Autodesk Inventor part; units mm, degrees
ref_plane "YZ Plane" through (0, 0, 0) normal (1, 0, 0) x (0, 1, 0)
ref_plane "XZ Plane" through (0, 0, 0) normal (0, 1, 0) x (-1, 0, 0)
ref_plane "XY Plane" through (0, 0, 0) normal (0, 0, 1) x (1, 0, 0)
sketch "Sketch1" plane through (0, 0, 0) normal (0, 1, 0) x (-1, 0, 0)
  line L0 (0, 0) -> (31, 0)
  line L1 (31, 0) -> (31, 4)
  line L2 (32, 5) -> (49, 5)
  line L3 (50, 4) -> (50, 0)
  line L4 (50, 0) -> (68, 0)
  line L5 (68, -52) -> (68, -85)
  line L6 (69, -86) -> (70, -86)
  line L7 (71, -87) -> (71, -272.1)
  line L8 (71, -272.1) -> (72.1718, -272.1)
  line L9 (72.8789, -272.3929) -> (74.7071, -274.2211)
  line L10 (75, -274.9282) -> (75, -284.1718)
  line L11 (74.7071, -284.8789) -> (72.8789, -286.7071)
  line L12 (72.1718, -287) -> (71, -287)
  line L13 (71, -287) -> (71, -293.6)
  line L14 (71, -293.6) -> (-26.8, -293.6)
  line L15 (-29.8, -290.6) -> (-29.8, -286)
  line L16 (0, 0) -> (0, 4)
  line L17 (-1, 5) -> (-18, 5)
  line L18 (-19, 4) -> (-19, 0)
  line L19 (-19, 0) -> (-24.8, 0)
  line L20 (-29.8, -5) -> (-29.8, -8.5)
  line L21 (-29.8, -8.5) -> (-37.8, -8.5)
  line L22 (-40.8, -11.5) -> (-40.8, -19.5)
  line L23 (-37.8, -22.5) -> (-7.9, -22.5)
  line L24 (-6.9, -23.5) -> (-6.9, -254)
  line L25 (-7.9, -255) -> (-26.8, -255)
  line L26 (-29.8, -258) -> (-29.8, -272)
  line L27 (-29.8, -272) -> (-37.8, -272)
  line L28 (-40.8, -275) -> (-40.8, -283)
  line L29 (-37.8, -286) -> (-29.8, -286)
  circle A0 centre (53.1, -11) radius 4
  circle A1 centre (-11.9, -11) radius 4
  circle A2 centre (53.1, -275) radius 4
  circle A3 centre (-11.9, -275) radius 4
  line L30 (69, -51) -> (70, -51)
  arc A4 (-18, 5) -> (-19, 4) centre (-18, 4) ccw
  arc A5 (0, 4) -> (-1, 5) centre (-1, 4) ccw
  arc A6 (32, 5) -> (31, 4) centre (32, 4) ccw
  arc A7 (50, 4) -> (49, 5) centre (49, 4) ccw
  arc A8 (-24.8, 0) -> (-29.8, -5) centre (-24.8, -5) ccw
  arc A9 (-7.9, -255) -> (-6.9, -254) centre (-7.9, -254) ccw
  arc A10 (-26.8, -255) -> (-29.8, -258) centre (-26.8, -258) ccw
  arc A11 (-37.8, -272) -> (-40.8, -275) centre (-37.8, -275) ccw
  arc A12 (-40.8, -283) -> (-37.8, -286) centre (-37.8, -283) ccw
  arc A13 (-40.8, -19.5) -> (-37.8, -22.5) centre (-37.8, -19.5) ccw
  arc A14 (-37.8, -8.5) -> (-40.8, -11.5) centre (-37.8, -11.5) ccw
  arc A15 (72.8789, -272.3929) -> (72.1718, -272.1) centre (72.1718, -273.1) ccw
  arc A16 (75, -274.9282) -> (74.7071, -274.2211) centre (74, -274.9282) ccw
  arc A17 (74.7071, -284.8789) -> (75, -284.1718) centre (74, -284.1718) ccw
  arc A18 (72.1718, -287) -> (72.8789, -286.7071) centre (72.1718, -286) ccw
  line L31 (71, -9.1) -> (72.1718, -9.1)
  line L32 (72.8789, -9.3929) -> (74.7071, -11.2211)
  line L33 (75, -11.9282) -> (75, -21.1718)
  line L34 (74.7071, -21.8789) -> (72.8789, -23.7071)
  line L35 (72.1718, -24) -> (71, -24)
  arc A19 (72.8789, -9.3929) -> (72.1718, -9.1) centre (72.1718, -10.1) ccw
  arc A20 (75, -11.9282) -> (74.7071, -11.2211) centre (74, -11.9282) ccw
  arc A21 (74.7071, -21.8789) -> (75, -21.1718) centre (74, -21.1718) ccw
  arc A22 (72.1718, -24) -> (72.8789, -23.7071) centre (72.1718, -23) ccw
  line L36 (71, -36.1) -> (72.1718, -36.1)
  line L37 (72.8789, -36.3929) -> (74.7071, -38.2211)
  line L38 (75, -38.9282) -> (75, -48.1718)
  line L39 (74.7071, -48.8789) -> (72.8789, -50.7071)
  line L40 (72.1718, -51) -> (71, -51)
  arc A23 (72.8789, -36.3929) -> (72.1718, -36.1) centre (72.1718, -37.1) ccw
  arc A24 (75, -38.9282) -> (74.7071, -38.2211) centre (74, -38.9282) ccw
  arc A25 (74.7071, -48.8789) -> (75, -48.1718) centre (74, -48.1718) ccw
  arc A26 (72.1718, -51) -> (72.8789, -50.7071) centre (72.1718, -50) ccw
  line L41 (71, -9.1) -> (71, -3)
  line L42 (71, -24) -> (71, -36.1)
  arc A27 (69, -51) -> (68, -52) centre (69, -52) ccw
  arc A28 (68, -85) -> (69, -86) centre (69, -85) ccw
  arc A29 (71, -87) -> (70, -86) centre (70, -87) ccw
  line L43 (71, -51) -> (70, -51)
  arc A30 (71, -3) -> (68, 0) centre (68, -3) ccw
  arc A31 (-6.9, -23.5) -> (-7.9, -22.5) centre (-7.9, -23.5) ccw
  arc A32 (-29.8, -290.6) -> (-26.8, -293.6) centre (-26.8, -290.6) ccw
  circle A33 centre (-36.8, -15.5) radius 2.15
  circle A34 centre (-36.8, -279) radius 2.15
  circle A35 centre (20.6, -6.5) radius 2.5
  point P0 (31, 5)
  point P1 (50, 5)
  point P2 (71, 0)
  point P3 (68, -86)
  point P4 (71, -86)
  point P5 (72.586, -272.1)
  point P6 (72.586, -287)
  point P7 (0, 5)
  point P8 (59, 0)
  point P9 (50, 2)
  point P10 (71, -5)
  point P11 (-22.85, -22.5)
  point P12 (-33.8, -8.5)
  point P13 (71.5859, -287)
  point P14 (71.8793, -10)
  point P15 (69.5, -51)
  point P16 (-21.9, 0)
  point P17 (71.5859, -24)
  point P18 (71.5859, -51)
  point P19 (69.5, -86)
  point P20 (-29.8, -6.75)
  point P21 (40.5, 5)
  dimension "d0" = 90
  dimension "d1" = 31
  dimension "d3" = 19
  dimension "d4" = 19
  dimension "d8" = 14
  dimension "d10" = 0
  dimension "d11" = 8
  dimension "d12" = 11
  dimension "d13" = 8
  dimension "d14" = 65
  dimension "d15" = 8
  dimension "d16" = 8
  dimension "d17" = 264
  dimension "d18" = 264
  dimension "d21" = 3
  dimension "d24" = 51
  dimension "d25" = 5
  dimension "d26" = 5
  dimension "d27" = 1
  dimension "d28" = 5
  dimension "d30" = 77.9
  dimension "d32" = 1
  dimension "d33" = 3
  dimension "d34" = 17
  dimension "d35" = 14
  dimension "d36" = 11
  dimension "d37" = 3
  dimension "d38" = 22.5
  dimension "d39" = 33.9
  dimension "d40" = 3
  dimension "d41" = 11
  dimension "d42" = 4
  dimension "d43" = 14.9
  dimension "d44" = 6.6
  dimension "d45" = 1.586
  dimension "d46" = 135
  dimension "d47" = 1.586
  dimension "d48" = 135
  dimension "d49" = 1
  dimension "d50" = 14.9
  dimension "d51" = 135
  dimension "d52" = 135
  dimension "d53" = 1
  dimension "d54" = 14.9
  dimension "d55" = 135
  dimension "d56" = 135
  dimension "d57" = 1
  dimension "d58" = 9.1
  dimension "d59" = 12.1
  dimension "d61" = 1
  dimension "d62" = 35
  dimension "d63" = 100.8
  dimension "d64" = 38.6
  dimension "d67" = 3
  dimension "d68" = 1
  dimension "d69" = 3
  dimension "d70" = 232.5
  dimension "d71" = 27.5
  dimension "d74" = 293.6
  dimension "d75" = 185.1
  dimension "d76" = 4.3
  dimension "d77" = 4
  dimension "d78" = 7
  dimension "d79" = 4
extrude "Extrusion1" add sketch "Sketch1" along normal blind 5 contours L0 L1 A6 L2 A7 L3 L4 A30 L41 L31 A19 L32 A20 L33 A21 L34 A22 L35 L42 L36 A23 L37 A24 L38 A25 L39 A26 L40 L43 L30 A27 L5 A28 L6 A29 L7 L8 A15 L9 A16 L10 A17 L11 A18 L12 L13 L14 A32 L15 L29 A12 L28 A11 L27 L26 A10 L25 A9 L24 A31 L23 A13 L22 A14 L21 L20 A8 L19 L18 A4 L17 A5 L16 | A33 | A34 | A35
extrude "Extrusion2" cut sketch "Sketch1" along normal blind 5 contours A33 | A34 | A35
fillet "Fillet1" radius 3 1 edges at (-71, 2.5, -293.6)
thread "Thread1"
thread "Thread2"
thread "Thread3"
thread "Thread4"
properties part number "21-30-220-B2"
The listing builds one solid part. Answer for the finished solid, in the listing's coordinates (mm). A direction names the side the tool comes from. Coordinates: 2 decimals unless noted, no trailing zeros. Loops run counter-clockwise (first coordinate to the right, second up) from the corner with the lowest first, then second, coordinate; pieces in that order, holes last.
1) Determine the mould class of faces 1 (the face through (22, 2, 0)), 2 (the face through (34, 2, -286)), 3 (the face through (10.054, 2.465, -271.451)) for opening direction Z: pulls with the +Z half, pulls with the -Z half, needs draft (parallel to the pull), parting line crosses it, or undercut.
2) Flat-ended cylindrical pins translate along their axes: pin 1 Ø1.5 at (y, z) = (2.5, -33) entering from -X; pin 2 Ø10 at (x, z) = (16.5, -40.5) entering from +Y; pin 3 Ø0.8 at (x, y) = (-69.5, 3) entering from +Z; pin 4 Ø0.9 at (x, y) = (-71.5, 2.5) entering from -Z. Find the tip coordinate at first contact, or state that the pin passes through.
3) Find section A-A on x = -53.1. Write down the section's boundary in (y, z), then the cut area to 3 significant figures.
4) Find section C-C on y = 1.8. Give the number of separate pieces and of enclosed holes in the cut face, then the cut area to 3 significant figures.
5) A tool of negligible diameter and unlimited length cuts with its end or side. For faces 4 (the face through (34, 2, -272)), 5 (the face through (-52.233, 2.465, -271.095)), 6 (the face through (40.8, 2, -15)), 7 (the face through (-71, 2, -30)), 8 (the face through (-71, 2, -6)), from which of +Z, -Z, +X, -X, +Y, -Y can it reach the whole face along a straight path? Write none if from no direction.
6) Find section B-B on z = -212. Write down the section's boundary in (x, y).
7) Find the intervals of material crossed by L1, parallel to Z at x = 36.8, y = 3.75; L2, parallel to Z at x = -53.1, y = 3.75; L3, parallel to X at y = 2, z = -275, in increasing order.
Values:
1. face 1: pulls with the +Z half
1. face 2: pulls with the -Z half
1. face 3: undercut
2. pin 1: stops at x = -71
2. pin 2: passes through
2. pin 3: stops at z = -0.21
2. pin 4: stops at z = -287
3. outline: (0, -293.6) - (5, -293.6) - (5, -279) - (0, -279) - close; (0, -271) - (5, -271) - (5, -15) - (0, -15) - close; (0, -7) - (5, -7) - (5, 0) - (0, 0) - close
3. area: 1,390 mm2
4. separate pieces: 1
4. enclosed holes: 7
4. area: 24,600 mm2
5. face 4: +X, +Y, -Y
5. face 5: +Y, -Y
5. face 6: +Z, -Z, +X, +Y, -Y
5. face 7: -X, +Y, -Y
5. face 8: +Z, -X, +Y, -Y
6. outline: (-71, 0) - (6.9, 0) - (6.9, 5) - (-71, 5) - close
7. L1: z = -286 to -281.15, -276.85 to -272, -22.5 to -17.65, -13.35 to -8.5
7. L2: z = -293.6 to -279, -271 to -15, -7 to 0
7. L3: x = -75 to -57.1, -49.1 to 7.9, 15.9 to 40.8
